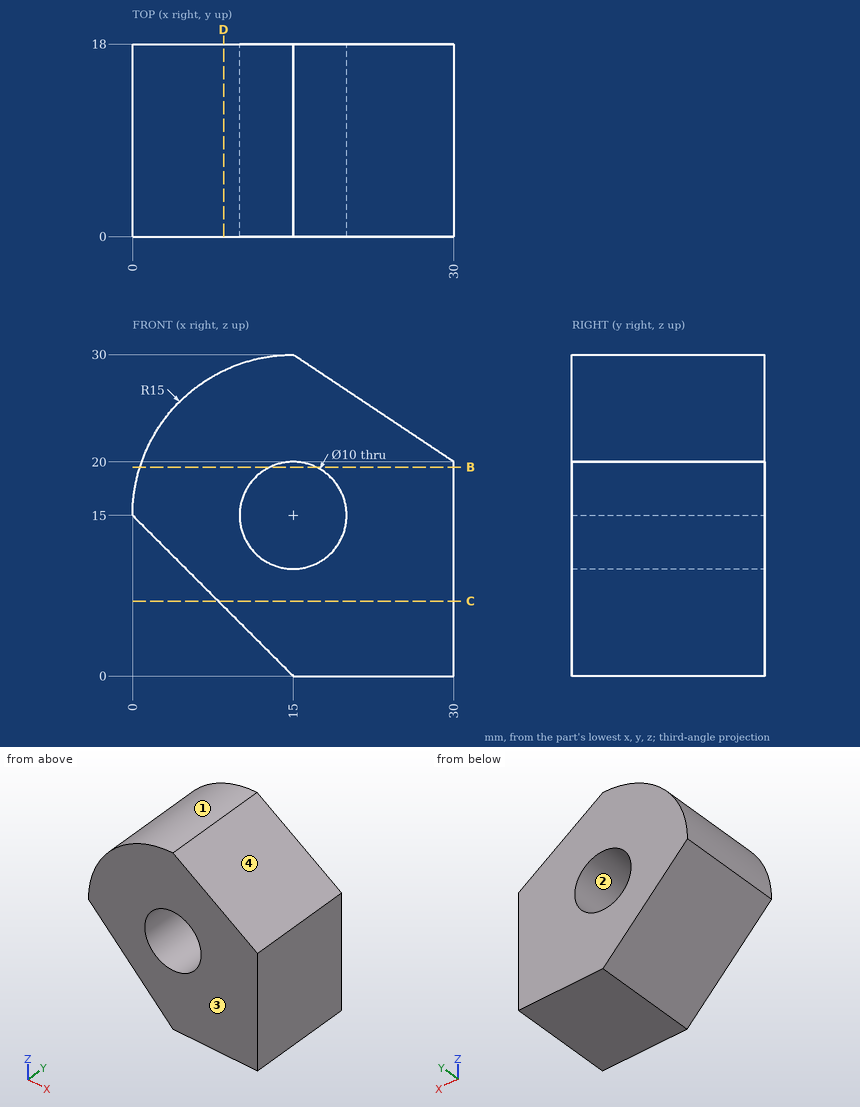
Check sheet for the drawn part. Datum: minimum x, y, z corner. Units: mm. Round coordinates to 2 decimals unless told otherwise and drop trailing zeros. Loops run counter-clockwise (first coordinate to the right, second up) from the corner with the lowest first, then second, coordinate; pieces in that order, holes last. Notation, with made-up numbers: (30, -22) - (56, -22) arc R37 cw to (56, 17) - close; hole circle Ø2 at (66, 87.5). An arc over 180 degrees is marked (long way). Write each question's results on one line, items separated by ' | '. Start each with the question number.
Q1. Release check for a two-part mould opening along X. For the marked faces 1, 2, 3 and 4 record: +X half, -X half, draft (parallel to the pull), parting line (faces both ways), or undercut.
Q2. Gauge pin test, flat ends, axial feed: P1, Ø2, axis at y = 11.5, z = 23, coming from the +X side; P2, Ø1, axis at y = 14, z = 24, coming from the -X side. Record the tip position at first contact, or that the pin passes through.
Q3. Cross-section at B-B on z = 19.5. Enter the section's corners in (x, y), and give its area (3 significant figures).
Q4. Cross-section at D-D on x = 8.5. Enter the section's corners in (y, z).
Q5. Cross-section at C-C on z = 7. Enter the section's corners in (x, y), and give its area (3 significant figures).
Q6. Thickness scan on line 1 (X direction, y = 12.5, z = 18.5); line 2 (Z direction, x = 13.5, y = 3); line 3 (X direction, y = 16, z = 11). Record the ranges inside material, lowest first. Write a range as [from, to].
Answers below:
1) face 1: -X half | face 2: undercut | face 3: draft | face 4: +X half
2) P1: stops at x = 27 | P2: stops at x = 2.64
3) outline: (0.69, 0) - (12.82, 0) - (12.82, 18) - (0.69, 18) - close; (17.18, 0) - (30, 0) - (30, 18) - (17.18, 18) - close | area: 449 mm²
4) outline: (0, 6.5) - (18, 6.5) - (18, 28.52) - (0, 28.52) - close
5) outline: (8, 0) - (30, 0) - (30, 18) - (8, 18) - close | area: 396 mm²
6) line 1: x = [0.41, 11.43], [18.57, 30] | line 2: z = [1.5, 10.23], [19.77, 29.92] | line 3: x = [4, 12], [18, 30]
